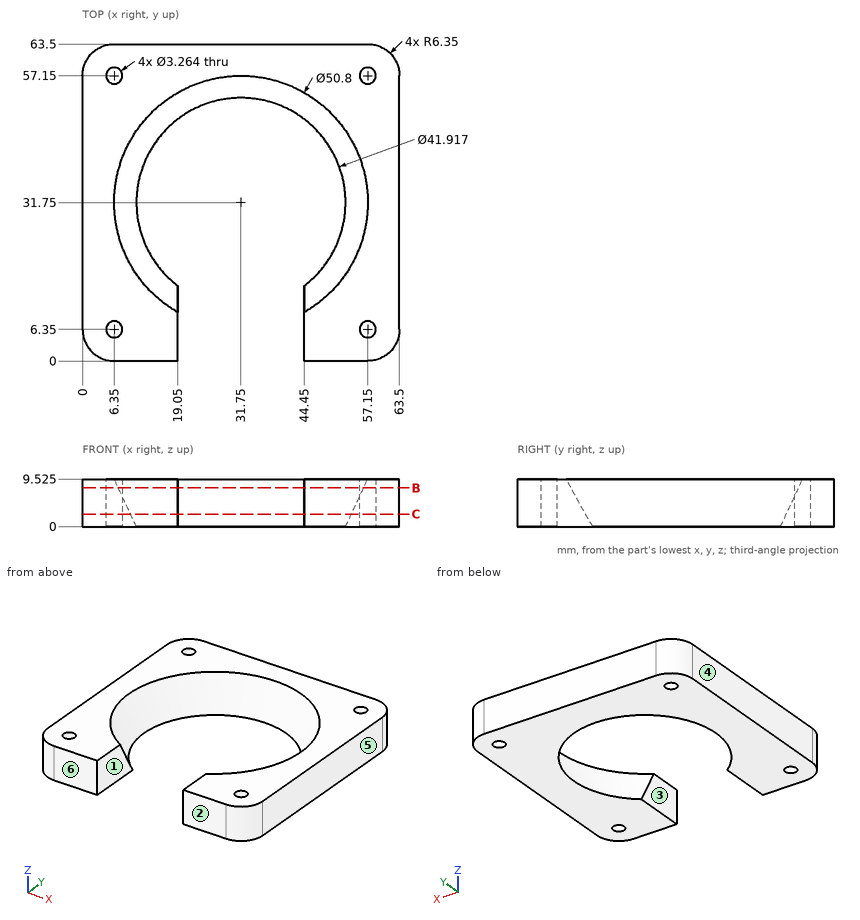
The figure shows three views and two pictorial views of one solid part (mm, origin at its lowest corner). Answer the questions. A direction names the side the tool comes from. Coordinates: 2 decimals unless noted, no trailing zeros. Loops run counter-clockwise (first coordinate to the right, second up) from the corner with the lowest first, then second, coordinate; pieces in that order, holes last.
1) Determine the mould class of the marked faces 3, 4, 5 and 6 for opening direction X: pulls with the +X half, pulls with the -X half, needs draft (parallel to the pull), parting line crosses it, or undercut.
2) A tool of negligible diameter and unlimited length cuts with its end or side. For the marked faces 1 and 2, from which of +Z, -Z, +X, -X, +Y, -Y can it reach the whole face along a straight path? Write none if from no direction.
3) Find section C-C on z = 2.5. Write down the section's boundary in (x, y).
4) Flat-ended cylindrical pins translate along their axes: pin 1 Ø3 at (x, y) = (33, 51) entering from +Z; pin 2 Ø4 at (x, z) = (31, 4) entering from -Y (3 decimals). Find the tip coordinate at first contact, or state that the pin passes through.
5) Find section B-B on z = 7.75. Write down the section's boundary in (x, y).
6) Find the intervals of material crossed by L1, parallel to Y at x = 57, z = 6.25 (3 decimals); L2, parallel to X at y = 9, z = 4, in increasing order.
Values:
1. face 3: undercut
1. face 4: pulls with the -X half
1. face 5: pulls with the +X half
1. face 6: needs draft
2. face 1: +Z, -Z, -Y
2. face 2: +Z, -Z, +X, -X, -Y
3. outline: (0, 6.35) arc R6.35 ccw to (6.35, 0) - (19.05, 0) - (19.05, 13.63) arc R22.12 cw (long way) to (44.45, 13.63) - (44.45, 0) - (57.15, 0) arc R6.35 ccw to (63.5, 6.35) - (63.5, 57.15) arc R6.35 ccw to (57.15, 63.5) - (6.35, 63.5) arc R6.35 ccw to (0, 57.15) - close; hole circle Ø3.26 at (6.35, 6.35); hole circle Ø3.26 at (6.35, 57.15); hole circle Ø3.26 at (57.15, 6.35); hole circle Ø3.26 at (57.15, 57.15)
4. pin 1: passes through
4. pin 2: stops at y = 53.625
5. outline: (0, 6.35) arc R6.35 ccw to (6.35, 0) - (19.05, 0) - (19.05, 10.71) arc R24.57 cw (long way) to (44.45, 10.71) - (44.45, 0) - (57.15, 0) arc R6.35 ccw to (63.5, 6.35) - (63.5, 57.15) arc R6.35 ccw to (57.15, 63.5) - (6.35, 63.5) arc R6.35 ccw to (0, 57.15) - close; hole circle Ø3.26 at (6.35, 6.35); hole circle Ø3.26 at (6.35, 57.15); hole circle Ø3.26 at (57.15, 6.35); hole circle Ø3.26 at (57.15, 57.15)
6. L1: y = 0 to 4.725, 7.975 to 55.525, 58.775 to 63.5
6. L2: x = 0 to 19.05, 44.45 to 63.5
